For this review, use the dimensioned drawing (mm, ordinates from the lowest corner) and the shaded views. A direction names the side the tool comes from. Give positions to 0.01 mm unless a question says otherwise; leave off trailing zeros. Loops run counter-clockwise (first coordinate to the right, second up) from the corner with the lowest first, then second, coordinate; pieces in that order, holes last. Notation, with made-up numbers: M 13.25,40.5 L 22.25,40.5 A15 cw 22.25,45.5 Z; hole C 24.25,60.5 d7. An arc over 180 degrees is marked long. Use CSV: the item, a comma, the result in double quotes.
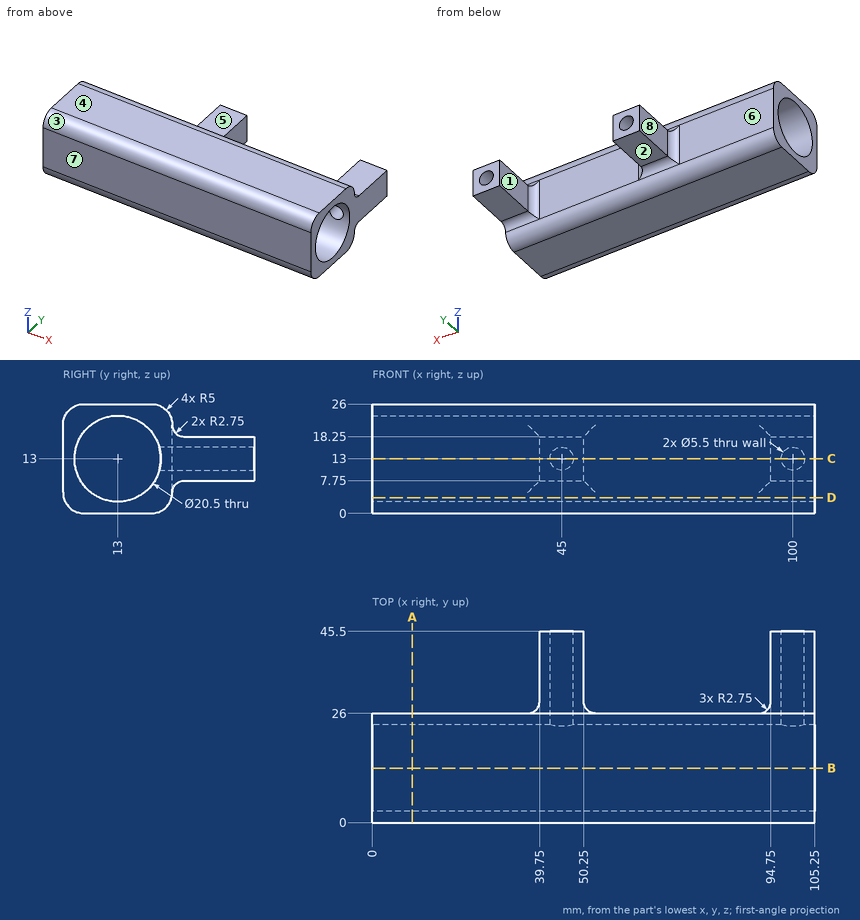
(1) Machinability: for the marked faces 1, 2, 3, 4 and 5, which of the approach directions +Z, -Z, +X, -X, +Y, -Y give a long, thin tool a straight path to every point of the face, cutting with its end or side? Answer none if there is none.
A:
face 1,"+Z, -Z, +Y"
face 2,"-Z, +X, -X, +Y"
face 3,"+Z, +X, -X, -Y"
face 4,"+Z, +X, -X, +Y, -Y"
face 5,"+Z, +X, -X, +Y"
(2) We need section A-A on x = 9.5. State the section outline as (y, z) points.
A:
outline,"M 0,5 A5 ccw 5,0 L 21,0 A5 ccw 26,5 L 26,21 A5 ccw 21,26 L 5,26 A5 ccw 0,21 Z; hole C 13,13 d20.5"
(3) We need section B-B on y = 13. State the section outline as (x, z) points, then the cut area to 3 significant figures.
A:
outline,"M 0,0 L 105.25,0 L 105.25,2.75 L 0,2.75 Z; M 0,23.25 L 105.25,23.25 L 105.25,26 L 0,26 Z"
area,"579 mm²"
(4) The part is to be moulded in two halves that separate along X. For the marked faces 6, 7 and 8, say which applies: released by +X, released by -X, zero draft, split by the parting line, or undercut.
A:
face 6,"zero draft"
face 7,"zero draft"
face 8,"released by -X"
(5) Clearance check with flat-ended pins moving along their axes: P1, Ø3.5, axis at x = 100, z = 13, coming from the +Y side; P2, Ø1.5, axis at y = 21, z = 8, coming from the -X side; P3, Ø8.5, axis at x = 102.5, y = 34.5, coming from the -Z side; P4, Ø11.5, axis at y = 41, z = 11, coming from the -X side. State where each tip first meets the part, or that it passes through.
A:
P1,"y = 2.9"
P2,"through"
P3,"z = 7.75"
P4,"x = 39.75"
(6) We need section C-C on z = 13. State the section outline as (x, y) points.
A:
outline,"M 0,0 L 105.25,0 L 105.25,2.75 L 0,2.75 Z; M 0,23.25 L 42.25,23.25 L 42.25,45.5 L 39.75,45.5 L 39.75,28.75 A2.75 cw 37,26 L 0,26 Z; M 47.75,23.25 L 97.25,23.25 L 97.25,45.5 L 94.75,45.5 L 94.75,28.75 A2.75 cw 92,26 L 53,26 A2.75 cw 50.25,28.75 L 50.25,45.5 L 47.75,45.5 Z; M 102.75,23.25 L 105.25,23.25 L 105.25,45.5 L 102.75,45.5 Z"
(7) We need section D-D on z = 3.75. State the section outline as (x, y) points, then the cut area to 3 significant figures.
A:
outline,"M 0,0.16 L 105.25,0.16 L 105.25,8.58 L 0,8.58 Z; M 0,17.42 L 105.25,17.42 L 105.25,25.84 L 0,25.84 Z"
area,"1,770 mm²"
(8) Wall thickness on line 1 along X through (y, z) = (40.25, 13); line 2 along Y through (x, z) = (29, 13); line 3 along X through (y, z) = (41.5, 16.5): over which ranges is each line inside the solid? List them lowest first. Write a range as [from, to].
A:
line 1,"[39.75, 42.25], [47.75, 50.25], [94.75, 97.25], [102.75, 105.25]"
line 2,"[0, 2.75], [23.25, 26]"
line 3,"[39.75, 50.25], [94.75, 105.25]"
